Here's the drawing with two shaded views (mm, measured from the low corner). I have some questions. A direction names the side the tool comes from. Give positions to 0.01 mm unless a question says otherwise; leave off trailing zeros. Write each loop counter-clockwise with the first axis right and the second up, starting at its lowest first coordinate (ties: lowest second). Pieces come first, ordered by that corner, then holes.
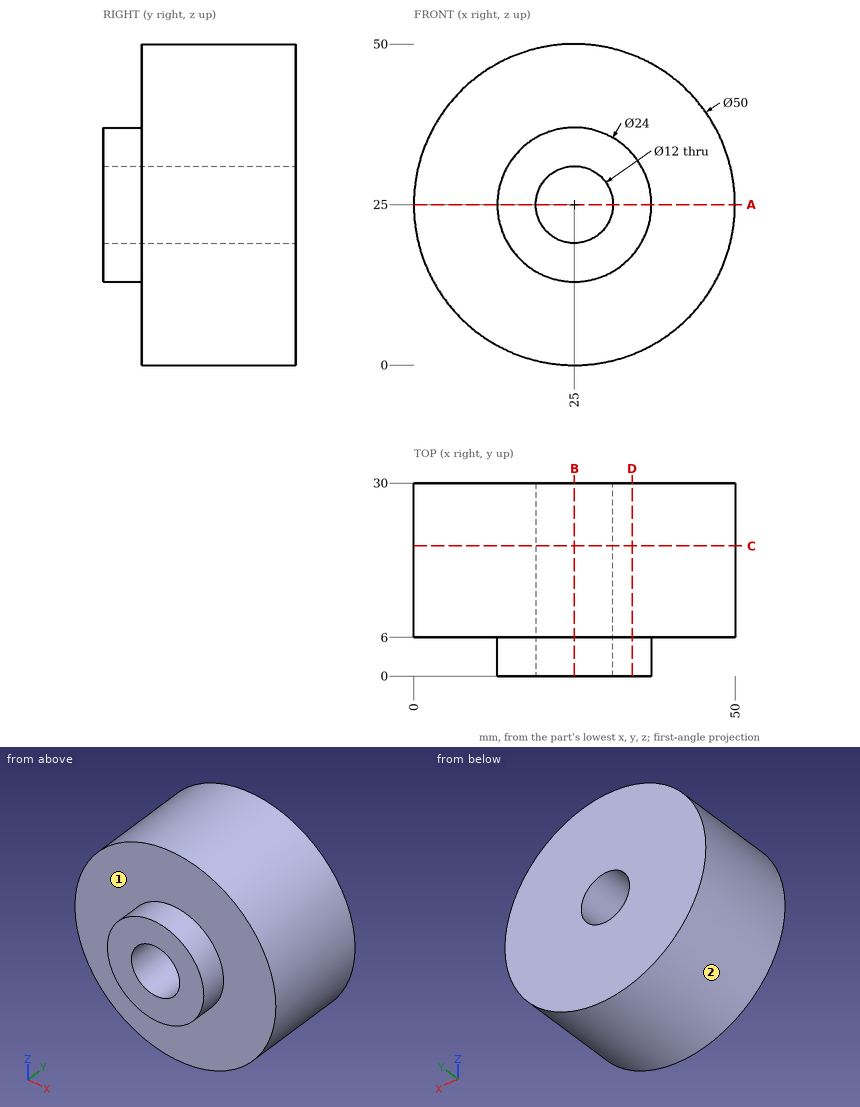
(1) For the marked faces 1 and 2, which set-ups out of +Z, -Z, +X, -X, +Y, -Y let a thin tool reach every point of the face, with its end or its side?
Returned:
face 1: -Y
face 2: +Y, -Y
(2) Imagine slicing it at D-D, the plane x = 34. Write out the boundary of the cut face in (y, z), plus the area to 3 significant figures.
Returned:
outline: (0, 17.06) - (6, 17.06) - (6, 1.68) - (30, 1.68) - (30, 48.32) - (6, 48.32) - (6, 32.94) - (0, 32.94) - close
area: 1,210 mm2
(3) If I drill on L1, parallel to Z at x = 25, y = 20.25; L2, parallel to Y at x = 34, z = 35; L3, parallel to Z at x = 21, y = 10.5, over which ranges is the centre line in solid material (lowest first)?
Returned:
L1: z = 0 to 19, 31 to 50
L2: y = 6 to 30
L3: z = 0.32 to 20.53, 29.47 to 49.68
(4) Will these pins go through, and if not, where does the flat tip stop? P1, Ø6, axis at x = 28, y = 10.5, coming from the -Z side; P2, Ø10, axis at y = 15.5, z = 6.5, coming from the -X side; P3, Ø2, axis at x = 22.5, y = 23.5, coming from the +Z side.
Returned:
P1: stops at z = 0
P2: stops at x = 3.96
P3: stops at z = 49.95
(5) Imagine slicing it at B-B, the plane x = 25. Write out the boundary of the cut face in (y, z).
Returned:
outline: (0, 13) - (6, 13) - (6, 0) - (30, 0) - (30, 19) - (0, 19) - close; (0, 31) - (30, 31) - (30, 50) - (6, 50) - (6, 37) - (0, 37) - close
(6) Imagine slicing it at A-A, the plane z = 25. Write out the boundary of the cut face in (x, y), plus the area to 3 significant figures.
Returned:
outline: (0, 6) - (13, 6) - (13, 0) - (19, 0) - (19, 30) - (0, 30) - close; (31, 0) - (37, 0) - (37, 6) - (50, 6) - (50, 30) - (31, 30) - close
area: 984 mm2
(7) Imagine slicing it at C-C, the plane y = 20.25. Write out the boundary of the cut face in (x, z), plus the area to 3 significant figures.
Returned:
outline: circle Ø50 at (25, 25); hole circle Ø12 at (25, 25)
area: 1,850 mm2
